For this review, take the finished solid that the model builds, in its own axes (mm). A direction names the side the tool comes from. Coordinates: 2 decimals unless noted, no trailing zeros. Loops run counter-clockwise (first coordinate to the right, second up) from the corner with the lowest first, then second, coordinate; pieces in that order, holes last.
1. Machinability: for faces 4 (the face through (-16, 3.398, 28)), 5 (the face through (18, 11, -18)), which of the approach directions +Z, -Z, +X, -X, +Y, -Y give a long, thin tool a straight path to every point of the face, cutting with its end or side? Answer none if there is none.
2. Take a section at B-B, the plane x = 0. State the section outline as (y, z) points, then the cut area to 3 significant figures.
3. Mouldability with a two-part tool opening along X and no side actions: class faces 1 (the face through (-37.95, 7.25, 3.06)), 2 (the face through (18, 0, -18)), 3 (the face through (-45.636, 5.423, -59.517)) as pulls with the +X half, pulls with the -X half, needs draft (parallel to the pull), parting line crosses it, or undercut.
4. Take a section at C-C, the plane y = 9. State the section outline as (x, z) points, then the cut area to 3 significant figures.
5. Take a section at A-A, the plane z = 0. State the section outline as (x, y) points.
6. To check wall thickness, follow probe 1 along X at (y, z) = (6, 0); probe 2 along Z at (x, y) = (0.5, 1.75) (3 decimals); probe 3 along X at (y, z) = (6, -26). State the ranges of each line that lie inside material, in increasing order.
7. Clearance check with flat-ended pins moving along their axes: P1, Ø4, axis at x = 34, z = -1, coming from the +Y side; P2, Ø4, axis at y = 1.5, z = 10, coming from the +X side; P3, Ø3, axis at x = 53.5, z = 20.5, coming from the -Y side; P4, Ø6, axis at y = 3, z = 22.5, coming from the +X side. State where each tip first meets the part, or that it passes through.
8. Take a section at D-D, the plane x = -17.5. State the section outline as (y, z) points.
```python
from build123d import *

# Parameters (mm, degrees)
SKETCH1_R             = 75
BOSS_EXTRUDE1_DEPTH   = 11
SKETCH2_R             = 25
CUT_EXTRUDE1_DEPTH    = 107.6348911
SKETCH3_R             = 6.621835616
CUT_EXTRUDE2_DEPTH    = 7.602484
CIRPATTERN1_START     = 3.397515695
CIRPATTERN1_OUTLINE_R = 6.621835616
CIRPATTERN1_DEPTH     = 7.602484305


# Read off the part's stored shape, not the designer's step: CirPattern1
with BuildPart() as part:
    # Sketch1 → Boss-Extrude1 (new body)
    with BuildSketch(Plane(origin=(0, 0, 0), x_dir=(1, 0, 0), z_dir=(0, 1, 0))):
        with Locations(Location((0, 0, 0), (0, 0, 270))):
            Circle(SKETCH1_R)
    extrude(amount=BOSS_EXTRUDE1_DEPTH)

    # Sketch2 → Cut-Extrude1 (cut, through all)
    with BuildSketch(Plane(origin=(0, 0, 0), x_dir=(1, 0, 0), z_dir=(0, 1, 0))):
        with Locations(Location((0, 0, 0), (0, 0, 270))):
            Circle(SKETCH2_R)
    extrude(amount=CUT_EXTRUDE1_DEPTH, mode=Mode.SUBTRACT)

    # Sketch3 → Cut-Extrude2 (cut)
    with BuildSketch(Plane(origin=(0, 11, 0), x_dir=(1, 0, 0), z_dir=(0, 1, 0))):
        with Locations(Location((-32.077977474, 0, 0), (0, 0, 270))):
            Circle(SKETCH3_R)
    extrude(amount=-CUT_EXTRUDE2_DEPTH, mode=Mode.SUBTRACT)

    # CirPattern1 outline → CirPattern1 (cut)
    with BuildSketch(Plane(origin=(0, 0, 0), x_dir=(1, 0, 0), z_dir=(0, 1, 0)).offset(CIRPATTERN1_START)):
        with Locations((-16.038988737, -27.780343394)):
            Circle(CIRPATTERN1_OUTLINE_R)
        with Locations((16.038988737, -27.780343394)):
            Circle(CIRPATTERN1_OUTLINE_R)
        with Locations((32.077977474, 0)):
            Circle(CIRPATTERN1_OUTLINE_R)
        with Locations((16.038988737, 27.780343394)):
            Circle(CIRPATTERN1_OUTLINE_R)
        with Locations((-16.038988737, 27.780343394)):
            Circle(CIRPATTERN1_OUTLINE_R)
    extrude(amount=CIRPATTERN1_DEPTH, mode=Mode.SUBTRACT)


solid = part.part
```
Results list:
1. face 4: +Y
1. face 5: +Z, -Z, +X, -X, +Y
2. outline: (0, -75) - (11, -75) - (11, -25) - (0, -25) - close; (0, 25) - (11, 25) - (11, 75) - (0, 75) - close
2. area: 1,100 mm2
3. face 1: undercut
3. face 2: needs draft
3. face 3: parting line crosses it
4. outline: circle Ø150 at (0, 0); hole circle Ø13.24 at (-32.08, 0); hole circle Ø50 at (0, 0); hole circle Ø13.24 at (-16.04, -27.78); hole circle Ø13.24 at (-16.04, 27.78); hole circle Ø13.24 at (16.04, -27.78); hole circle Ø13.24 at (16.04, 27.78); hole circle Ø13.24 at (32.08, 0)
4. area: 14,900 mm2
5. outline: (-75, 0) - (-25, 0) - (-25, 11) - (-25.46, 11) - (-25.46, 3.4) - (-38.7, 3.4) - (-38.7, 11) - (-75, 11) - close; (25, 0) - (75, 0) - (75, 11) - (38.7, 11) - (38.7, 3.4) - (25.46, 3.4) - (25.46, 11) - (25, 11) - close
6. probe 1: x = -75 to -38.7, -25.46 to -25, 25 to 25.46, 38.7 to 75
6. probe 2: z = -74.998 to -24.995, 24.995 to 74.998
6. probe 3: x = -70.35 to -22.42, -9.66 to 9.66, 22.42 to 70.35
7. P1: stops at y = 3.4
7. P2: stops at x = 74.57
7. P3: stops at y = 0
7. P4: stops at x = 72.42
8. outline: (0, -72.93) - (11, -72.93) - (11, -34.24) - (3.4, -34.24) - (3.4, -21.32) - (11, -21.32) - (11, -17.85) - (0, -17.85) - close; (0, 17.85) - (11, 17.85) - (11, 21.32) - (3.4, 21.32) - (3.4, 34.24) - (11, 34.24) - (11, 72.93) - (0, 72.93) - close
